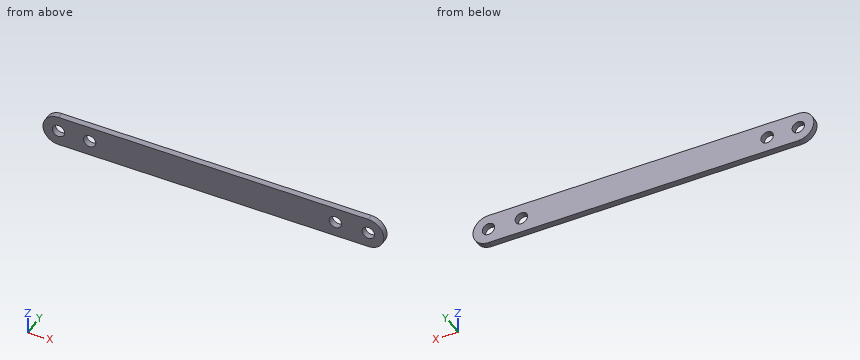
```python
from build123d import *

# Parameters (mm, degrees)
SKETCH_1_R          = 2.3
EXTRUDE_1_DEPTH     = 2
SKETCH_2_R          = 2.445702399
SKETCH_2_R_2        = 2
EXTRUDE_2_DEPTH     = 2
SKETCH_3_R          = 2.726249273
SKETCH_3_R_2        = 2
EXTRUDE_3_DEPTH     = 2
SKETCH_4_R          = 2
CUT_EXTRUDE_1_DEPTH = 2


with BuildPart() as part:
    # 草图1 → 凸台-拉伸1 (new body)
    with BuildSketch(Plane(origin=(0, 0, 0), x_dir=(1, 0, 0), z_dir=(0, 1, 0))):
        with BuildLine():
            Line((0, 5), (100, 5))
            ThreePointArc((100, 5), (105, 0), (100, -5))
            Line((100, -5), (0, -5))
            ThreePointArc((0, -5), (-5, 0), (0, 5))
        make_face()
        with Locations(Location((0, 0, 0), (0, 0, 270))):
            Circle(SKETCH_1_R, mode=Mode.SUBTRACT)
        with Locations(Location((100, 0, 0), (0, 0, 270))):
            Circle(SKETCH_1_R, mode=Mode.SUBTRACT)
    extrude(amount=EXTRUDE_1_DEPTH)

    # 草图2 → 凸台-拉伸2 (add)
    with BuildSketch(Plane(origin=(0, 2, 0), x_dir=(1, 0, 0), z_dir=(0, 1, 0))):
        Circle(SKETCH_2_R)
        with Locations(Location((0, 0, 0), (0, 0, 270))):
            Circle(SKETCH_2_R_2, mode=Mode.SUBTRACT)
    extrude(amount=-EXTRUDE_2_DEPTH)

    # 草图3 → 凸台-拉伸3 (add)
    with BuildSketch(Plane(origin=(0, 2, 0), x_dir=(1, 0, 0), z_dir=(0, 1, 0))):
        with Locations((100, 0)):
            Circle(SKETCH_3_R)
        with Locations(Location((100, 0, 0), (0, 0, 270))):
            Circle(SKETCH_3_R_2, mode=Mode.SUBTRACT)
    extrude(amount=-EXTRUDE_3_DEPTH)

    # 草图4 → 切除-拉伸1 (cut)
    with BuildSketch(Plane(origin=(0, 2, 0), x_dir=(1, 0, 0), z_dir=(0, 1, 0))):
        with Locations(Location((10.057445081, 0, 0), (0, 0, 270))):
            Circle(SKETCH_4_R)
        with Locations(Location((89.366430164, 0, 0), (0, 0, 270))):
            Circle(SKETCH_4_R)
    extrude(amount=-CUT_EXTRUDE_1_DEPTH, mode=Mode.SUBTRACT)


solid = part.part
```
Could you check a few things on this model? Use its own coordinates, in mm. Coordinates: 2 decimals unless noted, no trailing zeros. Write each loop counter-clockwise with the first axis right and the second up, starting at its lowest first coordinate (ties: lowest second). Pieces come first, ordered by that corner, then holes. Notation, with made-up numbers: (-6, -27.75) -> (21, -27.75) arc R20 cw to (21, -23.75) -> close; hole circle Ø7 at (-13.75, 14.25). An arc over 180 degrees is marked (long way). Write item = value, one per line. Start each with the question number.
(1) I want a section at B-B (y = 0.95). Please give me the cut outline in (x, z), plus the area to 3 significant figures.
(2) I want a section at A-A (z = 0). Please give me the cut outline in (x, y).
(3) I want a section at C-C (z = -4). Please give me the cut outline in (x, y), plus the area to 3 significant figures.
(4) I need wall thicknesses on line 1 (X direction, y = 1.6, z = 0.25); line 2 (X direction, y = 0.75, z = 0); line 3 (Z direction, x = 99, y = 1.3). Which ranges of each line are inside material? Lowest first, please. Write a range as [from, to].
Result set:
q1.outline = (0, -5) -> (100, -5) arc R5 ccw to (100, 5) -> (0, 5) arc R5 ccw to start; hole circle Ø4 at (0, 0); hole circle Ø4 at (10.06, 0); hole circle Ø4 at (89.37, 0); hole circle Ø4 at (100, 0)
q1.area = 1,030 mm2
q2.outline = (-5, 0) -> (-2, 0) -> (-2, 2) -> (-5, 2) -> close; (2, 0) -> (8.06, 0) -> (8.06, 2) -> (2, 2) -> close; (12.06, 0) -> (87.37, 0) -> (87.37, 2) -> (12.06, 2) -> close; (91.37, 0) -> (98, 0) -> (98, 2) -> (91.37, 2) -> close; (102, 0) -> (105, 0) -> (105, 2) -> (102, 2) -> close
q3.outline = (-3, 0) -> (103, 0) -> (103, 2) -> (-3, 2) -> close
q3.area = 212 mm2
q4.line_1 = [-4.99, -1.98], [1.98, 8.07], [12.04, 87.38], [91.35, 98.02], [101.98, 104.99]
q4.line_2 = [-5, -2], [2, 8.06], [12.06, 87.37], [91.37, 98], [102, 105]
q4.line_3 = [-5, -1.73], [1.73, 5]
